The model under review builds one solid part; all positions refer to its coordinate system, in mm. Coordinates: 2 decimals unless noted, no trailing zeros. Order: outer loops, then holes, each group sorted by start corner. A loop starts at its lowest first (then second) coordinate and runs counter-clockwise, first axis right, second up.
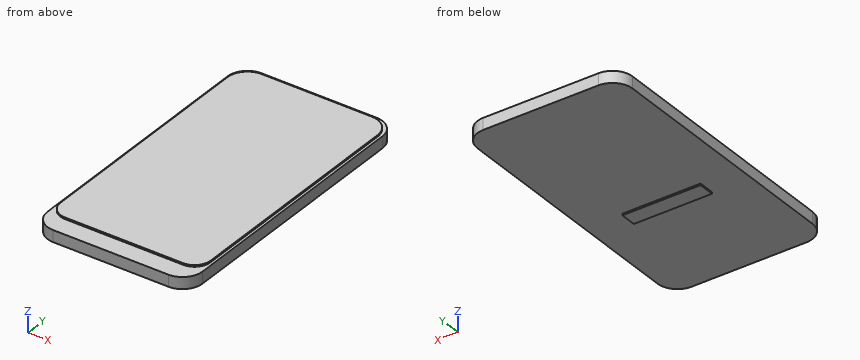
from build123d import *

# Parameters (mm, degrees)
BOSS_EXTRU_1_DEPTH = 1.46
BOSS_EXTRU_2_DEPTH = 0.15
BOSS_EXTRU_3_DEPTH = 0.2
CONG_1_R           = 0.01
CONTACTS_W         = 9.78910699
CONTACTS_H         = 1.999751064
BOSS_EXTRU_4_DEPTH = 0.2


with BuildPart() as part:
    # bordexterne → Boss.-Extru.1 (new body)
    with BuildSketch(Plane.XY):
        with BuildLine():
            Line((-7.154775328, -19.206177595), (7.239809861, -19.206177595))
            ThreePointArc((7.239809861, -19.206177595), (9.007576814, -18.473944548), (9.739809861, -16.706177595))
            Line((9.739809861, -16.706177595), (9.739809861, 14.688353392))
            ThreePointArc((9.739809861, 14.688353392), (9.007576814, 16.456120345), (7.239809861, 17.188353392))
            Line((7.239809861, 17.188353392), (-7.154775328, 17.188353392))
            ThreePointArc((-7.154775328, 17.188353392), (-8.922542281, 16.456120345), (-9.654775328, 14.688353392))
            Line((-9.654775328, 14.688353392), (-9.654775328, -16.706177595))
            ThreePointArc((-9.654775328, -16.706177595), (-8.922542281, -18.473944548), (-7.154775328, -19.206177595))
        make_face()
    extrude(amount=-BOSS_EXTRU_1_DEPTH)

    # surfaceutile → Boss.-Extru.2 (add)
    with BuildSketch(Plane.XY):
        with BuildLine():
            Line((-6.695, -16.175), (6.695, -16.175))
            ThreePointArc((6.695, -16.175), (8.109213562, -15.589213562), (8.695, -14.175))
            Line((8.695, -14.175), (8.695, 14.175))
            ThreePointArc((8.695, 14.175), (8.109213562, 15.589213562), (6.695, 16.175))
            Line((6.695, 16.175), (-6.695, 16.175))
            ThreePointArc((-6.695, 16.175), (-8.109213562, 15.589213562), (-8.695, 14.175))
            Line((-8.695, 14.175), (-8.695, -14.175))
            ThreePointArc((-8.695, -14.175), (-8.109213562, -15.589213562), (-6.695, -16.175))
        make_face()
    extrude(amount=BOSS_EXTRU_2_DEPTH)

    # bord2 → Boss.-Extru.3 (add)
    with BuildSketch(Plane.XY):
        with BuildLine():
            Line((-7.395, -16.825), (7.395, -16.825))
            ThreePointArc((7.395, -16.825), (8.809213562, -16.239213562), (9.395, -14.825))
            Line((9.395, -14.825), (9.395, 14.325))
            ThreePointArc((9.395, 14.325), (8.662766953, 16.092766953), (6.895, 16.825))
            Line((6.895, 16.825), (-6.895, 16.825))
            ThreePointArc((-6.895, 16.825), (-8.662766953, 16.092766953), (-9.395, 14.325))
            Line((-9.395, 14.325), (-9.395, -14.825))
            ThreePointArc((-9.395, -14.825), (-8.809213562, -16.239213562), (-7.395, -16.825))
        make_face()
    extrude(amount=BOSS_EXTRU_3_DEPTH)

    # Congé1
    cong_1_edges = [part.edges().sort_by_distance(p)[0] for p in [
        (8.809213562, -16.239213562, 0.2),
        (9.395, -0.25, 0.2),
        (8.662766953, 16.092766953, 0.2),
        (0, 16.825, 0.2),
        (-8.662766953, 16.092766953, 0.2),
        (-9.395, -0.25, 0.2),
        (-8.809213562, -16.239213562, 0.2),
        (0, -16.825, 0.2),
    ]]
    fillet(cong_1_edges, radius=CONG_1_R)

    # contacts → Boss.-Extru.4 (add)
    with BuildSketch(Plane(origin=(0, 0, -1.46), x_dir=(-1, 0, 0), z_dir=(0, 0, -1))):
        with Locations((-0.066948969, -4.908420558)):
            Rectangle(CONTACTS_W, CONTACTS_H)
    extrude(amount=BOSS_EXTRU_4_DEPTH)


solid = part.part
(1) Wall thickness on line 1 (Z direction, x = -0.5, y = 14); line 2 (Z direction, x = 9.25, y = -16.5); line 3 (X direction, y = -3, z = 0.1) (3 decimals): over which ranges is each line inside the solid? List them lowest first.
(2) Consider section D-D (x = 5.5). Give the boundary of the cut face in (y, z) (3 decimals), then the cut area to 3 significant figures.
(3) Insertion check: pin 1 Ø10 at (x, y) = (4.5, -14) entering from -Z. The pin has a flat end and moves straight along its axis. Give the tip position at first contact, or say it passes through.
(4) Consider section B-B (x = 0.75). Give the boundary of the cut face in (y, z) (3 decimals).
(5) Consider section A-A (y = 10). Give the boundary of the cut face in (x, z) (3 decimals), then the cut area to 3 significant figures.
Findings:
1. line 1: z = -1.46 to 0.2
1. line 2: z = -1.46 to 0
1. line 3: x = -9.395 to 9.395
2. outline: (-19.206, -1.46) - (17.188, -1.46) - (17.188, 0) - (16.825, 0) - (16.825, 0.19) arc R0.01 ccw to (16.815, 0.2) - (-16.815, 0.2) arc R0.01 ccw to (-16.825, 0.19) - (-16.825, 0) - (-19.206, 0) - close
2. area: 59.9 mm2
3. pin 1: stops at z = -1.46
4. outline: (-19.206, -1.46) - (-5.908, -1.46) - (-5.908, -1.66) - (-3.909, -1.66) - (-3.909, -1.46) - (17.188, -1.46) - (17.188, 0) - (16.825, 0) - (16.825, 0.19) arc R0.01 ccw to (16.815, 0.2) - (-16.815, 0.2) arc R0.01 ccw to (-16.825, 0.19) - (-16.825, 0) - (-19.206, 0) - close
5. outline: (-9.655, -1.46) - (9.74, -1.46) - (9.74, 0) - (9.395, 0) - (9.395, 0.19) arc R0.01 ccw to (9.385, 0.2) - (-9.385, 0.2) arc R0.01 ccw to (-9.395, 0.19) - (-9.395, 0) - (-9.655, 0) - close
5. area: 32.1 mm2
